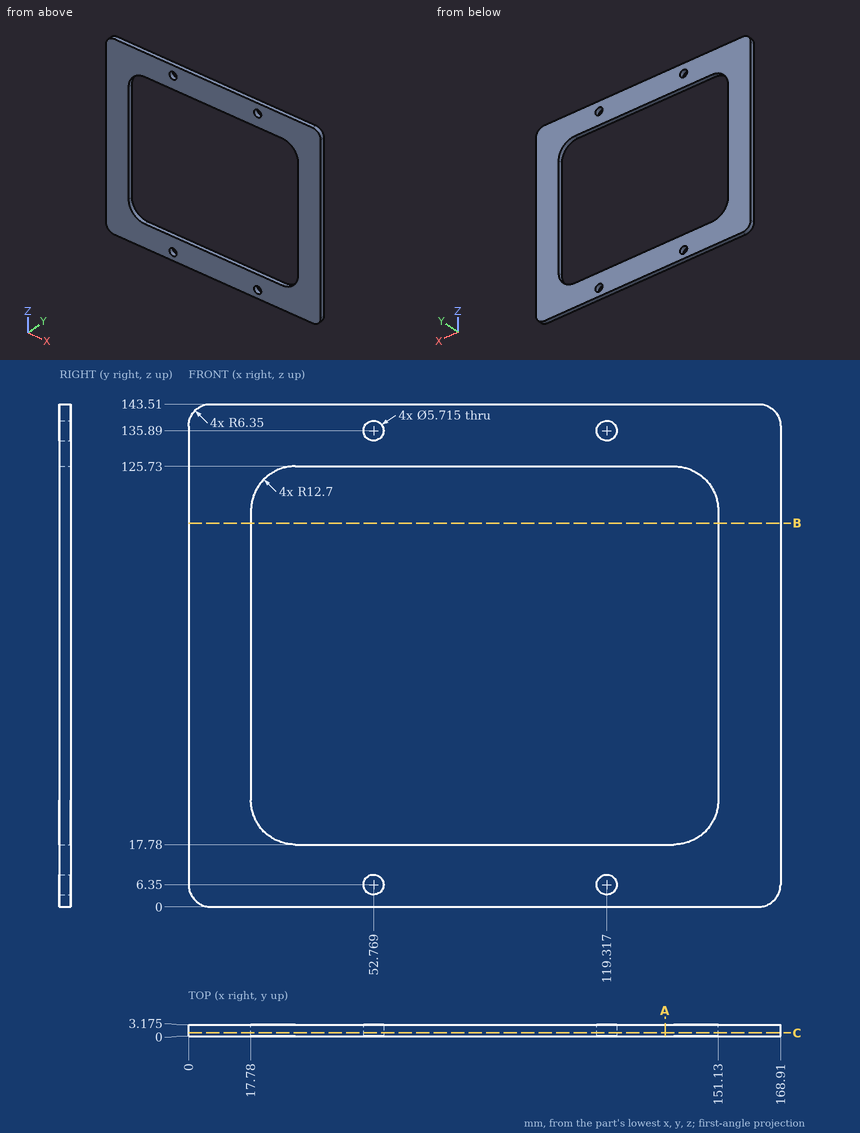
Geometry check sheet. Reference: drawing and pictorial views, mm from the part's lowest x, y, z. Give positions to 0.01 mm unless a question says otherwise; leave off trailing zeros. Order: outer loops, then holes, each group sorted by start corner. A loop starts at its lowest first (then second) coordinate and runs counter-clockwise, first axis right, second up. Notation, with made-up numbers: M -21.5,83 L 20.5,83 A25 cw 20.5,96 Z; hole C 71.25,44 d9. An arc over 180 degrees is marked long. Use one line per item in the form item = value. Start each with the question number.
Q1. Scan lines: line 1 along X through (y, z) = (2.3, 6.35) (1 decimal); line 2 along X through (y, z) = (2.8, 88); line 3 along Z through (x, y) = (62.5, 1.3). Record each from-to range of solid material in increasing order. Write a range as [from, to].
Q2. Section check B-B (z = 109.5). Enter the section's corners in (x, y) (1 decimal), then the cut area to 3 significant figures.
Q3. Section check A-A (x = 136). Enter the section's corners in (y, z) (1 decimal).
Q4. Section check C-C (y = 0.9). Count the separate pieces of the cut face and the enclosed holes in it, then the cut area to 3 significant figures.
Evaluation:
q1.line_1 = [0, 49.9], [55.6, 116.5], [122.2, 168.9]
q1.line_2 = [0, 17.78], [151.13, 168.91]
q1.line_3 = [0, 17.78], [125.73, 143.51]
q2.outline = M 0,0 L 17.8,0 L 17.8,3.2 L 0,3.2 Z; M 151.1,0 L 168.9,0 L 168.9,3.2 L 151.1,3.2 Z
q2.area = 113 mm2
q3.outline = M 0,0 L 3.2,0 L 3.2,17.8 L 0,17.8 Z; M 0,125.7 L 3.2,125.7 L 3.2,143.5 L 0,143.5 Z
q4.separate_pieces = 1
q4.enclosed_holes = 5
q4.area = 9,850 mm2
